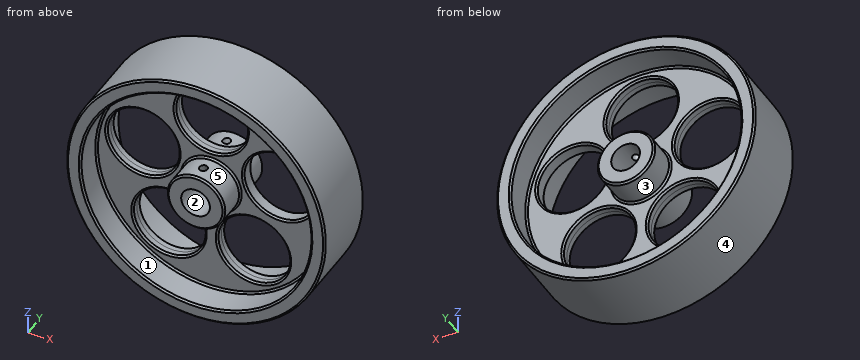
from build123d import *

# Parameters (mm, degrees)
F2_R      = 15.875
F3_DEPTH  = 25.4
F7_R      = 1.7272
F8_DEPTH  = 12.5777076509
F9_R      = 1.7272
F10_DEPTH = 12.5777076509
F11_SIZE  = 0.79375


with BuildPart() as f1:
    # F0 (on Right) → F1 (revolve)
    with BuildSketch(Plane.YZ):
        Polygon((-16.256, 12.7), (-16.256, 6.35), (16.256, 6.35), (16.256, 12.7), (3.175, 12.7), (3.175, 50.8), (16.256, 50.8), (16.256, 57.15), (-16.256, 57.15), (-16.256, 50.8), (-3.175, 50.8), (-3.175, 12.7), align=None)
    revolve(axis=Axis((0, 1.0807417785, 0), (0, 1, 0)))

    # F2 (on Front) → F3 (cut, symmetric)
    with BuildSketch(Plane.XZ):
        with Locations((0, 31.75)):
            Circle(F2_R)
        with Locations((-30.1960443924, 9.8112895714)):
            Circle(F2_R)
        with Locations((-18.6621817603, -25.6862895714)):
            Circle(F2_R)
        with Locations((18.6621817603, -25.6862895714)):
            Circle(F2_R)
        with Locations((30.1960443924, 9.8112895714)):
            Circle(F2_R)
    extrude(amount=F3_DEPTH, both=True, mode=Mode.SUBTRACT)

    # F7 (on line) → F8 (cut, up to face)
    with BuildSketch(Plane(origin=(0, -7.4394877579, 17.9605122421), x_dir=(1, 0, 0), z_dir=(0, 0.3826834324, -0.9238795325))):
        with Locations((0, 4.1158720071)):
            Circle(F7_R)
    extrude(amount=F8_DEPTH, mode=Mode.SUBTRACT)

    # F9 (on line) → F10 (cut, up to face)
    with BuildSketch(Plane(origin=(0, 7.4394877579, 17.9605122421), x_dir=(1, 0, 0), z_dir=(0, 0.3826834324, 0.9238795325))):
        with Locations((0, 4.1158720071)):
            Circle(F9_R)
    extrude(amount=-F10_DEPTH, mode=Mode.SUBTRACT)

    # F11
    f11_edges = [f1.edges().sort_by_distance(p)[0] for p in [
        (0, -16.256, -57.15),
        (0, 16.256, -57.15),
        (0, -16.256, -50.8),
        (0, -3.175, -50.8),
        (0, 16.256, -50.8),
        (0, 3.175, -50.8),
        (0, 16.256, -12.7),
        (0, 3.175, -12.7),
        (0, -16.256, -12.7),
        (0, -3.175, -12.7),
        (-15.875, -3.175, 31.75),
        (14.321044, -3.175, 9.81129),
        (2.787182, -3.175, -25.68629),
        (-34.537182, -3.175, -25.68629),
        (-46.071044, -3.175, 9.81129),
        (-15.875, 3.175, 31.75),
        (-46.071044, 3.175, 9.81129),
        (-34.537182, 3.175, -25.68629),
        (2.787182, 3.175, -25.68629),
        (14.321044, 3.175, 9.81129),
    ]]
    chamfer(f11_edges, length=F11_SIZE)


solid = f1.part
The model under review builds one solid part; all positions refer to its coordinate system, in mm. Face numbers are marked on the shaded views. A direction names the side the tool comes from. Give positions to 0.01 mm unless a question says otherwise; leave off trailing zeros. Loops run counter-clockwise (first coordinate to the right, second up) from the corner with the lowest first, then second, coordinate; pieces in that order, holes last. Notation, with made-up numbers: (-14, 41) -> (20, 41) arc R36 cw to (20, 75) -> close; hole circle Ø10 at (8.5, 6). An arc over 180 degrees is marked (long way). Write each question's results on one line, items separated by ' | '.
1) Take a section at A-A, the plane y = -13. Give the boundary of the cut face in (x, z), plus the area to 3 significant figures.
Conclusion:
outline: circle Ø114.3 at (0, 0); circle Ø25.4 at (0, 0); hole circle Ø101.6 at (0, 0); hole circle Ø12.7 at (0, 0) | area: 2,530 mm^2
2) Take a section at B-B, the plane z = 0. Count the separate pieces of the cut face and the enclosed holes in it, plus the area to 3 significant figures.
Conclusion:
separate pieces: 4 | enclosed holes: 0 | area: 988 mm^2
3) For line 1 along Z through (x, y) = (-10.5, -8); line 2 along Z through (x, y) = (-1, 5.5); line 3 along X through (y, z) = (6.5, -4), list the stretches that pass through material, from the lowest coordinate up. Write a range as from..to.
Conclusion:
line 1: z = -56.18..-49.7, -7.14..7.14, 49.7..56.18 | line 2: z = -57.14..-50.79, -12.66..-6.27, 6.27..12.66, 50.79..57.14 | line 3: x = -57.01..-50.64, -12.05..-4.93, 4.93..12.05, 50.64..57.01
4) Draft analysis for pull direction Z (two halves, no side actions). For the marked faces 4 and 5, state which applies: pulls with the +Z half, pulls with the -Z half, needs draft (parallel to the pull), parting line crosses it, or undercut.
Conclusion:
face 4: parting line crosses it | face 5: undercut
5) Insertion check: pin 1 Ø4 at (x, z) = (-43, 42) entering from +Y; pin 2 Ø1 at (x, z) = (22, -5) entering from +Y (3 decimals); pin 3 Ø12 at (x, y) = (-8.5, 8) entering from +Z; pin 4 Ø4 at (x, y) = (34, 11) entering from -Z. Each pin has a flat end and moves straight along its axis. Give the tip position at first contact, or say it passes through.
Conclusion:
pin 1: passes through | pin 2: stops at y = 3.175 | pin 3: stops at z = 57.1 | pin 4: stops at z = -47.35
6) Tool access review of the marked faces 1, 2 and 3: name each direction out of +Z, -Z, +X, -X, +Y, -Y from which nothing blocks a thin tool from reaching the whole face with its end or side.
Conclusion:
face 1: -Y | face 2: +Y, -Y | face 3: +Y
